Geometry: final body of the model. Coordinates: model frame, mm. A direction names the side the tool comes from. Give positions to 0.01 mm unless a question says otherwise; leave off trailing zeros. Write each loop counter-clockwise with the first axis right and the second up, starting at its lowest first coordinate (ties: lowest second). Pieces come first, ordered by that corner, then holes. Notation, with made-up numbers: (64.25, 58.25) - (80.25, 58.25) arc R31 ccw to (80.25, 83.25) - close; hole circle Ø7 at (-37, 60.5). An arc over 180 degrees is marked (long way). Use CSV: the item, a comma, the result in double quotes. Start each with the question number.
(1) Section A-A on y = 6.35. Output: boundary loops of the cut face in (x, z) (3 decimals), and give its area (3 significant figures).
(2) Section C-C on z = 137. Output: boundary loops of the cut face in (x, y) (3 decimals), and give its area (3 significant figures).
(3) First-contact query: pin 1 Ø7.5 at (y, z) = (-16, 89.5) entering from -X; pin 2 Ø10 at (x, z) = (4, 78.5) entering from -Y; pin 3 Ø1 at (x, y) = (6.5, 7.5) entering from -Z. Flat tips, straight axial feed; report the tip coordinate or a pass-through.
(4) Section D-D on x = 4.75. Output: boundary loops of the cut face in (y, z), and give its area (3 significant figures).
(5) Draft query along Y for faces 4 (the flat face through (4, 6, 50.8)), 5 (the flat face through (17, -25.4, 75)), 6 (the flat face through (-1.947, 6, 75)). Return one class per face: released by +Y, released by -Y, zero draft, split by the parting line, or undercut.
(6) Reachability of faces 1 (the flat face through (10.753, -13, 75)), 2 (the cylindrical face through (1.47, 7.57, 127.36)), 3 (the cylindrical face through (2.7, 9.03, 25.04)) from +Z, -Z, +X, -X, +Y, -Y: full face, straight path, thin tool, end or side. Return the list, or none.
(7) Line query: probe 1 along Z at (x, y) = (4.5, 8.5); probe 2 along X at (y, z) = (8.25, 76.2); probe 3 along Y at (x, z) = (10.25, 32). Output: solid intervals per line, ascending. Write a range as [from, to].
(8) Section B-B on z = 76.2. Output: boundary loops of the cut face in (x, y).
Autodesk Inventor part; units mm, degrees
ref_plane "YZ Plane" through (0, 0, 0) normal (1, 0, 0) x (0, 1, 0)
ref_plane "XZ Plane" through (0, 0, 0) normal (0, 1, 0) x (-1, 0, 0)
ref_plane "XY Plane" through (0, 0, 0) normal (0, 0, 1) x (1, 0, 0)
sketch "Sketch1" plane through (0, 0, 0) normal (0, 0, 1) x (1, 0, 0)
  line L0 (0, 0) -> (10.7529, 0)
  line L1 (10.7529, 0) -> (10.7529, -25.4)
  line L2 (10.7529, -25.4) -> (23.4529, -25.4)
  line L3 (23.4529, -25.4) -> (23.4529, 12.7)
  line L4 (23.4529, 12.7) -> (-1.9471, 12.7)
  line L5 (-1.9471, 12.7) -> (-1.9471, 0)
  line L6 (-1.9471, 0) -> (10.7529, 0)
  dimension "d0" = 25.4
  dimension "d1" = 12.7
  dimension "d2" = 12.7
  dimension "d3" = 12.7
extrude "Extrusion1" add sketch "Sketch1" along normal blind 152.4
sketch "Sketch2" plane through (-1.9471, 12.7, 0) normal (0, 1, 0) x (1, 0, 0)
  circle A0 centre (6.35, -76.2) radius 3.175
  line L0 (25.4, -152.4) -> (0, -152.4)
  line L1 (0, 0) -> (0, -152.4)
  point P0 (1.9471, 0)
  dimension "d6" = 6.35
  dimension "d7" = 76.2
  dimension "d8" = 6.35
extrude "Extrusion2" cut sketch "Sketch2" against normal blind 12.7
sketch "Sketch3" plane through (0, 0, 0) normal (0, 0, -1) x (-1, 0, 0)
  circle A0 centre (-4.4029, 6.35) radius 3.175
  line L0 (1.9471, 0) -> (-10.7529, 0)
  line L1 (1.9471, 12.7) -> (1.9471, 0)
  point P0 (0, 0)
  dimension "d11" = 6.35
  dimension "d12" = 6.35
  dimension "d13" = 6.35
extrude "Extrusion3" cut sketch "Sketch3" against normal blind 50.8
ref_plane "Work Plane1" through (-1.9471, 12.7, 76.2) normal (0, 0, -1) x (1, 0, 0)
mirror "Mirror1" about plane through (-1.9471, 12.7, 76.2) normal (0, 0, -1) of "Extrusion3"
properties part number "FuselageWingBoxJoint"
Check values:
1,outline,"(-1.947, 0) - (1.228, 0) - (1.228, 50.8) - (7.578, 50.8) - (7.578, 0) - (23.453, 0) - (23.453, 152.4) - (7.578, 152.4) - (7.578, 101.6) - (1.228, 101.6) - (1.228, 152.4) - (-1.947, 152.4) - close; hole circle Ø6.35 at (4.403, 76.2)"
1,area,"3,190 mm²"
2,outline,"(-1.947, 0) - (10.753, 0) - (10.753, -25.4) - (23.453, -25.4) - (23.453, 12.7) - (-1.947, 12.7) - close; hole circle Ø6.35 at (4.403, 6.35)"
2,area,"613 mm²"
3,pin 1,"stops at x = 10.75"
3,pin 2,"stops at y = 0"
3,pin 3,"stops at z = 50.8"
4,outline,"(0, 0) - (3.19, 0) - (3.19, 50.8) - (9.51, 50.8) - (9.51, 0) - (12.7, 0) - (12.7, 73.04) - (0, 73.04) - close; (0, 79.36) - (12.7, 79.36) - (12.7, 152.4) - (9.51, 152.4) - (9.51, 101.6) - (3.19, 101.6) - (3.19, 152.4) - (0, 152.4) - close"
4,area,"1,210 mm²"
5,face 4,"undercut"
5,face 5,"released by -Y"
5,face 6,"zero draft"
6,face 1,"+Z, -Z, -X, -Y"
6,face 2,"+Z"
6,face 3,"-Z"
7,probe 1,"z = [50.8, 73.03], [79.37, 101.6]"
7,probe 2,"x = [-1.95, 1.23], [7.58, 23.45]"
7,probe 3,"y = [0, 12.7]"
8,outline,"(-1.95, 0) - (1.23, 0) - (1.23, 12.7) - (-1.95, 12.7) - close; (7.58, 0) - (10.75, 0) - (10.75, -25.4) - (23.45, -25.4) - (23.45, 12.7) - (7.58, 12.7) - close"
